Verification items for this drawing (mm, ordinates from the low corner). Give positions to 0.01 mm unless a question says otherwise; leave off trailing zeros. Loops run counter-clockwise (first coordinate to the right, second up) from the corner with the lowest first, then second, coordinate; pieces in that order, holes last. Notation, with made-up numbers: (7.5, -11) -> (66.5, -11) arc R16 cw to (66.5, -1) -> close; hole circle Ø10 at (-22, -31). An arc over 180 degrees is marked (long way). Answer as a JSON object with one key per item and string values.
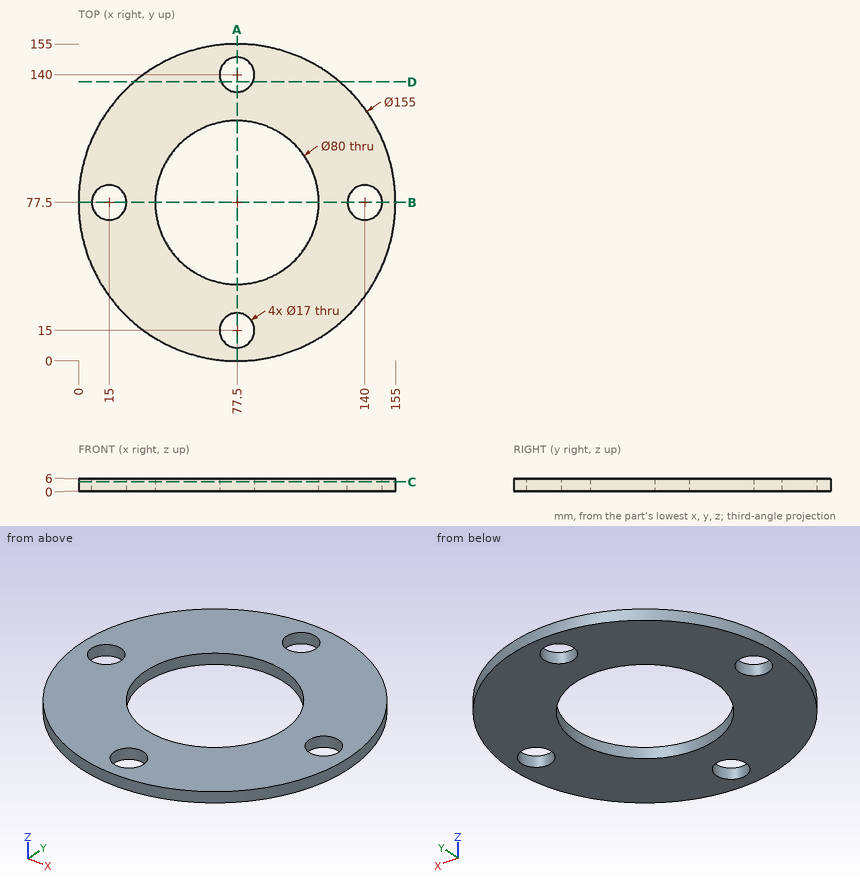
1) Section check D-D on y = 136.5. Record the cut outline in (x, z), plus the area to 3 significant figures.
Geometry check:
{"outline": "(27.25, 0) -> (69.75, 0) -> (69.75, 6) -> (27.25, 6) -> close; (85.25, 0) -> (127.75, 0) -> (127.75, 6) -> (85.25, 6) -> close", "area": "510 mm2"}
2) Material ranges on line 1 along Y through (x, z) = (77.5, 1.8); line 2 along X through (y, z) = (80.5, 0.35); line 3 along X through (y, z) = (106.5, 0.75), recorded low to high. Write a range as from..to.
Geometry check:
{"line 1": "y = 0..6.5, 23.5..37.5, 117.5..131.5, 148.5..155", "line 2": "x = 0.06..7.05, 22.95..37.61, 117.39..132.05, 147.95..154.94", "line 3": "x = 5.63..49.95, 105.05..149.37"}
3) Section check C-C on z = 4.55. Record the cut outline in (x, y), plus the area to 3 significant figures.
Geometry check:
{"outline": "circle Ø155 at (77.5, 77.5); hole circle Ø17 at (15, 77.5); hole circle Ø80 at (77.5, 77.5); hole circle Ø17 at (77.5, 15); hole circle Ø17 at (77.5, 140); hole circle Ø17 at (140, 77.5)", "area": "12,900 mm2"}
4) Depth check by flat-ended pin: P1, Ø2, axis at y = 58, z = 5.5, coming from the +X side; P2, Ø10, axis at x = 77.5, y = 140, coming from the -Z side (3 decimals); P3, Ø2, axis at y = 55, z = 1.5, coming from the -X side; P4, Ø1.5, axis at y = 78.5, z = 5, coming from the +X side. Enter the tip coordinate at first touch or a pass-through.
Geometry check:
{"P1": "stops at x = 152.76", "P2": "passes through", "P3": "stops at x = 3.04", "P4": "stops at x = 155"}
5) Section check A-A on x = 77.5. Record the cut outline in (y, z), plus the area to 3 significant figures.
Geometry check:
{"outline": "(0, 0) -> (6.5, 0) -> (6.5, 6) -> (0, 6) -> close; (23.5, 0) -> (37.5, 0) -> (37.5, 6) -> (23.5, 6) -> close; (117.5, 0) -> (131.5, 0) -> (131.5, 6) -> (117.5, 6) -> close; (148.5, 0) -> (155, 0) -> (155, 6) -> (148.5, 6) -> close", "area": "246 mm2"}
